from build123d import *

# Parameters (mm, degrees)
F0_R     = 25
F1_DEPTH = 300
F3_R     = 22.5
F4_DEPTH = 600


with BuildPart() as f1:
    # F0 (on Front) → F1 (new body)
    with BuildSketch(Plane.XZ):
        Circle(F0_R)
    extrude(amount=-F1_DEPTH)

    # F2: F1 across face


with BuildPart() as f1_1:
    add(f1.part)
    add(f1.part.mirror(Plane.XZ))

    # F3 (on face) → F4 (cut)
    with BuildSketch(Plane.XZ.offset(300)):
        Circle(F3_R)
    extrude(amount=-F4_DEPTH, mode=Mode.SUBTRACT)


solid = f1_1.part
Model file for the job. Use its own axes, mm. Round coordinates to 2 decimals unless told otherwise and drop trailing zeros. Loops run counter-clockwise (first coordinate to the right, second up) from the corner with the lowest first, then second, coordinate; pieces in that order, holes last.
1. Mould opens along X. For faces 1 (the flat face through (-22.34, 300, 3.82)), 2 (the cylindrical face through (10.382, -4.2, -19.961)) say: +X half, -X half, draft (parallel to the pull), parting line (faces both ways), or undercut.
Check values:
face 1: draft
face 2: undercut
2. Band-saw the part on A-A, the plane x = 0. List the corners of the cut face in (y, z).
Check values:
outline: (-300, -25) - (300, -25) - (300, -22.5) - (-300, -22.5) - close; (-300, 22.5) - (300, 22.5) - (300, 25) - (-300, 25) - close
3. Wall check: probe 1 along Z at (x, y) = (0, -146); probe 2 along Z at (x, y) = (9, 103.5); probe 3 along X at (y, z) = (165, 5.5). Give the ranges that are in metal, low to high.
Check values:
probe 1: z = -25 to -22.5, 22.5 to 25
probe 2: z = -23.32 to -20.62, 20.62 to 23.32
probe 3: x = -24.39 to -21.82, 21.82 to 24.39
4. Band-saw the part on B-B, the plane z = 0. List the corners of the cut face in (x, y).
Check values:
outline: (-25, -300) - (-22.5, -300) - (-22.5, 300) - (-25, 300) - close; (22.5, -300) - (25, -300) - (25, 300) - (22.5, 300) - close
5. Band-saw the part on C-C, the plane y = 29. List the corners of the cut face in (x, z), and give its area (3 significant figures).
Check values:
outline: circle Ø50 at (0, 0); hole circle Ø45 at (0, 0)
area: 373 mm2
6. Drop flat-ended pins along their axis: P1, Ø4, axis at y = -88.5, z = -8.5, coming from the -X side; P2, Ø10, axis at y = 236.5, z = -13.5, coming from the +X side; P3, Ø6, axis at y = -52.5, z = -6.5, coming from the -X side. Give the stop position or say it passes through.
Check values:
P1: stops at x = -24.14
P2: stops at x = 23.51
P3: stops at x = -24.75
